Autodesk Inventor part; units mm, degrees
ref_plane "YZ Plane" through (0, 0, 0) normal (1, 0, 0) x (0, 1, 0)
ref_plane "XZ Plane" through (0, 0, 0) normal (0, 1, 0) x (-1, 0, 0)
ref_plane "XY Plane" through (0, 0, 0) normal (0, 0, 1) x (1, 0, 0)
sketch "Esboço1" plane through (0, 0, 0) normal (1, 0, 0) x (0, 1, 0)
  line L0 (0, 0) -> (-3.2, 0)
  line L1 (-6, 0) -> (-6, 2)
  line L2 (-6, 2) -> (2, 2)
  line L3 (2, 2) -> (2, -42)
  line L4 (2, -42) -> (0, -42)
  line L5 (0, -42) -> (0, 0)
  line L6 (-6, 0) -> (-6, -2)
  line L7 (-6, -2) -> (-3.2, -2)
  line L8 (-3.2, -2) -> (-3.2, 0)
  dimension "d0" = 6
  dimension "d1" = 2
  dimension "d2" = 8
  dimension "d3" = 44
  dimension "d4" = 2
  dimension "d5" = 2.8
extrude "Extrusão1" add sketch "Esboço1" along normal blind 19
sketch "Esboço2" plane through (0, 2, 2) normal (0, 1, 0) x (1, 0, 0)
  line L0 (0, 44) -> (19, 44)
  line L1 (14.5, 44) -> (14.5, 36)
  line L2 (4.5, 36) -> (4.5, 44)
  line L3 (0, 44) -> (0, 0)
  line L4 (4.5, 36) -> (0, 36)
  line L5 (0, 36) -> (0, 44)
  line L6 (0, 44) -> (4.5, 44)
  line L7 (4.5, 44) -> (4.5, 36)
  line L8 (19, 44) -> (19, 0)
  line L9 (14.5, 36) -> (19, 36)
  line L10 (19, 36) -> (19, 44)
  line L11 (19, 44) -> (14.5, 44)
  line L12 (14.5, 44) -> (14.5, 36)
  point P0 (0, 2)
  point P1 (0, 36)
extrude "Extrusão2" cut sketch "Esboço2" against normal blind 19
fillet "Arredondamento1" radius 5 2 edges at (14.5, 1, -42) (4.5, 1, -42)
sketch "Esboço3" plane through (0, 2, 2) normal (0, 1, 0) x (1, 0, 0)
  circle A0 centre (9.5, 39) radius 1.5
  line L0 (14.5, 36) -> (14.5, 39)
  arc A1 (14.5, 39) -> (4.5, 39) centre (9.5, 39) ccw
  point P0 (0, 2)
  dimension "d14" = 3
  dimension "d15" = 5
  dimension "d16" = 0
extrude "Extrusão3" cut sketch "Esboço3" against normal blind 19
properties part number "tampa hc12"
Could you check a few things on this model? Use its own coordinates, in mm. A direction names the side the tool comes from. Round coordinates to 2 decimals unless told otherwise and drop trailing zeros. Write each loop counter-clockwise with the first axis right and the second up, starting at its lowest first coordinate (ties: lowest second). Pieces come first, ordered by that corner, then holes. Notation, with made-up numbers: (32.25, -32) - (48.25, -32) arc R9 cw to (48.25, -28) - close; hole circle Ø5 at (79.25, 82). An arc over 180 degrees is marked (long way). Put each result on its own line as item: value. Start each with the question number.
(1) Thinking about a two-plate mould opening in Y: for faces 1 (the flat face through (17, 1, -34)), 2 (the flat face through (9, -2, 0)), 3 (the flat face through (9, -6, 0)), which applies, released by +Y, released by -Y, zero draft, split by the parting line, or undercut?
(2) Will these pins go through, and if not, where does the flat tip stop? pin 1 (1 mm diameter, centred on x = 11.5, y = -1, fed in from -Z); pin 2 (0.8 mm diameter, centred on x = 6, y = -4, fed in from -Z); pin 3 (8 mm diameter, centred on x = 2.5, z = -13, fed in from -Y); pin 4 (2.5 mm diameter, centred on x = 9.5, z = -37, fed in from +Y).
(3) I want a section at D-D, the plane x = 6.5. Please give me the cut outline in (y, z), plus the area to 3 significant figures.
(4) I want a section at C-C, the plane y = -5. Please give me the cut outline in (x, z).
(5) I want a section at B-B, the plane z = -35. Please give me the cut outline in (x, y), plus the area to 3 significant figures.
(6) I need wall thicknesses on probe 1 along Z at (x, y) = (9.5, 0.4); probe 2 along X at (y, z) = (1.15, -37); probe 3 along Y at (x, z) = (1.25, -7). Which ranges of each line are inside material? Lowest first, please.
(7) For faces 4 (the flat face through (14.5, 1, -36)), 5 (the flat face through (9, -3.2, -1)), 6 (the cylindrical face through (9.175, 1.014, -35.536)), 7 (the flat face through (9, -5, -2)), 8 (the flat face through (4.5, 1, -35)), which set-ups out of +Z, -Z, +X, -X, +Y, -Y let a thin tool reach every point of the face, with its end or its side?
Here are the results:
1. face 1: zero draft
1. face 2: undercut
1. face 3: released by -Y
2. pin 1: stops at z = 0
2. pin 2: stops at z = -2
2. pin 3: stops at y = 0
2. pin 4: passes through
3. outline: (-6, -2) - (-3.2, -2) - (-3.2, 0) - (0, 0) - (0, -41) - (2, -41) - (2, 2) - (-6, 2) - close
3. area: 104 mm^2
4. outline: (0, -2) - (19, -2) - (19, 2) - (0, 2) - close
5. outline: (4.5, 0) - (14.5, 0) - (14.5, 2) - (4.5, 2) - close
5. area: 20.0 mm^2
6. probe 1: z = -42 to -38.5, -35.5 to 2
6. probe 2: x = 4.5 to 8, 11 to 14.5
6. probe 3: y = 0 to 2
7. face 4: -Z, +X, +Y, -Y
7. face 5: -Z, +X, -X
7. face 6: +Y, -Y
7. face 7: -Z, +X, -X, -Y
7. face 8: -Z, -X, +Y, -Y
